Design review of the part built by this model. Coordinates are the model's own, in mm. A direction names the side the tool comes from. Coordinates: 2 decimals unless noted, no trailing zeros. Write each loop counter-clockwise with the first axis right and the second up, starting at its lowest first coordinate (ties: lowest second). Pieces come first, ordered by that corner, then holes.
Q1. Mouldability with a two-part tool opening along X and no side actions: class faces 1 (the cylindrical face through (18.313, -7.593, 22.255)), 2 (the flat face through (-11, 0, 40)), 3 (the cylindrical face through (-13.73, -20.39, -1.34)) as pulls with the +X half, pulls with the -X half, needs draft (parallel to the pull), parting line crosses it, or undercut.
Q2. Take a section at D-D (y = 10.5). Give the boundary of the cut face in (x, z).
Q3. Take a section at B-B (z = 36). Give the boundary of the cut face in (x, y) (3 decimals), and give its area (3 significant figures).
Q4. Take a section at C-C (z = 16). Give the boundary of the cut face in (x, y) (3 decimals), and give its area (3 significant figures).
Q5. Take a section at A-A (y = 0). Give the boundary of the cut face in (x, z) (3 decimals), and give its area (3 significant figures).
Q6. Insertion check: pin 1 (10.5 mm diameter, centred on x = 0, y = 0, fed in from +Z); pin 2 (1.5 mm diameter, centred on x = -14.5, z = 8.5, fed in from +Y); pin 3 (8.5 mm diameter, centred on y = 3.5, z = 29.5, fed in from +X) (3 decimals); pin 4 (8.5 mm diameter, centred on x = 17.5, y = -17.5, fed in from +Z). Each pin has a flat end and moves straight along its axis. Give the tip position at first contact, or say it passes through.
Q7. For probe 1 along Z at (x, y) = (-4.5, 26.5); probe 2 along Y at (x, z) = (0, -3); probe 3 along X at (y, z) = (0.5, 4), list the stretches that pass through material, from the lowest coordinate up.
Q8. Machinability: for faces 4 (the cylindrical face through (3.25, -0.07, 33.94)), 5 (the flat face through (0, 25, 5)), 6 (the flat face through (0, 11, 34)), which of the approach directions +Z, -Z, +X, -X, +Y, -Y give a long, thin tool a straight path to every point of the face, cutting with its end or side? Answer none if there is none.
```python
from build123d import *

# Parameters (mm, degrees)
CROQUIS1_R                 = 35.5
CROQUIS1_R_2               = 3.25
SALIENTE_EXTRUIR1_DEPTH    = 5
CROQUIS9_R                 = 19.825
CROQUIS9_R_2               = 3.25
SALIENTE_EXTRUIR4_DEPTH    = 35
CORTAR_EXTRUIR4_DEPTH      = 36.5
CORTAR_EXTRUIR4_DEPTH_BACK = 36.5
CROQUIS11_R                = 35.5
CROQUIS11_R_2              = 3.25
SALIENTE_EXTRUIR5_DEPTH    = 7.5
CORTAR_EXTRUIR5_DEPTH      = 7.5
CORTAR_EXTRUIR7_DEPTH      = 13.5
CORTAR_EXTRUIR8_REACH      = 49.5
CROQUIS16_R                = 4.75


with BuildPart() as part:
    # Croquis1 → Saliente-Extruir1 (new body)
    with BuildSketch(Plane.XY):
        Circle(CROQUIS1_R)
        Circle(CROQUIS1_R_2, mode=Mode.SUBTRACT)
    extrude(amount=SALIENTE_EXTRUIR1_DEPTH)

    # Croquis9 → Saliente-Extruir4 (add)
    with BuildSketch(Plane.XY.offset(5)):
        Circle(CROQUIS9_R)
        Circle(CROQUIS9_R_2, mode=Mode.SUBTRACT)
    extrude(amount=SALIENTE_EXTRUIR4_DEPTH)

    # Croquis10 → Cortar-Extruir4 (cut, two sides)
    with BuildSketch(Plane(origin=(0, 0, 0), x_dir=(1, 0, 0), z_dir=(0, 1, 0))) as cortar_extruir4_sk:
        with BuildLine():
            Line((0, -29), (0, -40))
            Line((0, -40), (-6, -40))
            Line((-6, -40), (-6, -23))
            ThreePointArc((-6, -23), (4.242640687, -18.757359313), (0, -29))
        make_face()
    extrude(amount=CORTAR_EXTRUIR4_DEPTH, mode=Mode.SUBTRACT)
    extrude(cortar_extruir4_sk.sketch, amount=-CORTAR_EXTRUIR4_DEPTH_BACK, mode=Mode.SUBTRACT)

    # Croquis11 → Saliente-Extruir5 (add)
    with BuildSketch(Plane(origin=(0, 0, 0), x_dir=(-1, 0, 0), z_dir=(0, 0, -1))):
        Circle(CROQUIS11_R)
        Circle(CROQUIS11_R_2, mode=Mode.SUBTRACT)
    extrude(amount=SALIENTE_EXTRUIR5_DEPTH)

    # Croquis13 → Cortar-Extruir5 (cut)
    with BuildSketch(Plane.XY.offset(5)):
        with BuildLine():
            Line((-20, -29.330018752), (20, -29.330018752))
            ThreePointArc((20, -29.330018752), (0, -35.5), (-20, -29.330018752))
        make_face()
    extrude(amount=-CORTAR_EXTRUIR5_DEPTH, mode=Mode.SUBTRACT)

    # Croquis15 → Cortar-Extruir7 (cut, through all)
    with BuildSketch(Plane.XY.offset(5)):
        with BuildLine():
            Line((20, -29.330018752), (-20, -29.330018752))
            ThreePointArc((-20, -29.330018752), (0, -35.5), (20, -29.330018752))
        make_face()
    extrude(amount=-CORTAR_EXTRUIR7_DEPTH, mode=Mode.SUBTRACT)

    # Croquis16 → Cortar-Extruir8 (cut, up to next)
    with BuildSketch(Plane(origin=(0, 0, -7.5), x_dir=(-1, 0, 0), z_dir=(0, 0, -1)), mode=Mode.PRIVATE) as cortar_extruir8_sk1:
        with Locations((17.500892834, -17.500892834)):
            Circle(CROQUIS16_R)
    cortar_extruir8_tool1 = extrude(cortar_extruir8_sk1.sketch, amount=-CORTAR_EXTRUIR8_REACH, mode=Mode.PRIVATE) & part.part
    add(cortar_extruir8_tool1.solids().sort_by_distance((-17.500893, -17.500893, -7.5))[0], mode=Mode.SUBTRACT)
    # Croquis16 → Cortar-Extruir8 (cut, up to next)
    with BuildSketch(Plane(origin=(0, 0, -7.5), x_dir=(-1, 0, 0), z_dir=(0, 0, -1)), mode=Mode.PRIVATE) as cortar_extruir8_sk2:
        with Locations((-17.500892834, -17.500892834)):
            Circle(CROQUIS16_R)
    cortar_extruir8_tool2 = extrude(cortar_extruir8_sk2.sketch, amount=-CORTAR_EXTRUIR8_REACH, mode=Mode.PRIVATE) & part.part
    add(cortar_extruir8_tool2.solids().sort_by_distance((17.500893, -17.500893, -7.5))[0], mode=Mode.SUBTRACT)
    # Croquis16 → Cortar-Extruir8 (cut, up to next)
    with BuildSketch(Plane(origin=(0, 0, -7.5), x_dir=(-1, 0, 0), z_dir=(0, 0, -1)), mode=Mode.PRIVATE) as cortar_extruir8_sk3:
        with Locations((-17.500892834, 17.500892834)):
            Circle(CROQUIS16_R)
    cortar_extruir8_tool3 = extrude(cortar_extruir8_sk3.sketch, amount=-CORTAR_EXTRUIR8_REACH, mode=Mode.PRIVATE) & part.part
    add(cortar_extruir8_tool3.solids().sort_by_distance((17.500893, 17.500893, -7.5))[0], mode=Mode.SUBTRACT)
    # Croquis16 → Cortar-Extruir8 (cut, up to next)
    with BuildSketch(Plane(origin=(0, 0, -7.5), x_dir=(-1, 0, 0), z_dir=(0, 0, -1)), mode=Mode.PRIVATE) as cortar_extruir8_sk4:
        with Locations((17.500892834, 17.500892834)):
            Circle(CROQUIS16_R)
    cortar_extruir8_tool4 = extrude(cortar_extruir8_sk4.sketch, amount=-CORTAR_EXTRUIR8_REACH, mode=Mode.PRIVATE) & part.part
    add(cortar_extruir8_tool4.solids().sort_by_distance((-17.500893, 17.500893, -7.5))[0], mode=Mode.SUBTRACT)


solid = part.part
```
Response:
1. face 1: parting line crosses it
1. face 2: needs draft
1. face 3: undercut
2. outline: (-33.91, -7.5) - (33.91, -7.5) - (33.91, 5) - (16.82, 5) - (16.82, 40) - (0, 40) - (0, 29) arc R6 cw (long way) to (-6, 23) - (-6, 40) - (-16.82, 40) - (-16.82, 5) - (-33.91, 5) - close
3. outline: (-6, -18.895) - (-6, 18.895) arc R19.825 ccw to start; (0, -19.825) arc R19.825 ccw to (0, 19.825) - (0, 3.25) arc R3.25 cw to (0, -3.25) - close
3. area: 984 mm2
4. outline: circle Ø39.65 at (0, 0); hole circle Ø6.5 at (0, 0)
4. area: 1,200 mm2
5. outline: (-35.5, -7.5) - (-3.25, -7.5) - (-3.25, 17.956) arc R6 cw to (-6, 23) - (-6, 40) - (-19.825, 40) - (-19.825, 5) - (-35.5, 5) - close; (3.25, -7.5) - (35.5, -7.5) - (35.5, 5) - (19.825, 5) - (19.825, 40) - (3.25, 40) - (3.25, 28.044) arc R6 cw to (3.25, 17.956) - close
5. area: 1,890 mm2
6. pin 1: stops at z = 40
6. pin 2: stops at y = 14.28
6. pin 3: stops at x = 19.825
6. pin 4: passes through
7. probe 1: z = -7.5 to 5
7. probe 2: y = -29.33 to -3.25, 3.25 to 35.5
7. probe 3: x = -35.5 to -3.21, 3.21 to 35.5
8. face 4: +Z, -Z
8. face 5: +Z
8. face 6: +Z, +Y, -Y
